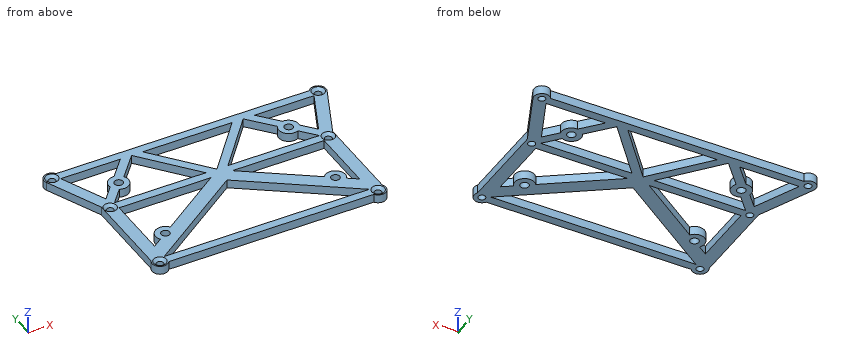
```python
from build123d import *

# Parameters (mm, degrees)
SKETCH1_R           = 1.25
BOSS_EXTRUDE1_DEPTH = 3
CHAMFER1_SIZE       = 1
SKETCH2_R           = 3.5
BOSS_EXTRUDE2_DEPTH = 3
SKETCH2_3_R         = 1.5
CUT_EXTRUDE1_DEPTH  = 3


with BuildPart() as part:
    # Sketch1 → Boss-Extrude1 (new body)
    with BuildSketch(Plane.XY):
        with BuildLine():
            Line((6.173773471, 33.368208058), (-2.509184891, 52.727938114))
            ThreePointArc((-2.509184891, 52.727938114), (-1.316660917, 56.267635348), (2.304886114, 55.353323017))
            Line((2.304886114, 55.353323017), (91.695113886, 55.353323017))
            ThreePointArc((91.695113886, 55.353323017), (95.316660917, 56.267635348), (96.509184891, 52.727938114))
            Line((96.509184891, 52.727938114), (87.826226529, 33.368208058))
            Line((87.826226529, 33.368208058), (87.826226529, 1.466686789))
            ThreePointArc((87.826226529, 1.466686789), (86.983381771, -2.315616229), (83.195113886, -1.5))
            Line((83.195113886, -1.5), (10.804886114, -1.5))
            ThreePointArc((10.804886114, -1.5), (7.016618229, -2.315616229), (6.173773471, 1.466686789))
            Line((6.173773471, 1.466686789), (6.173773471, 33.368208058))
        make_face()
        with Locations((0, 53.853323017)):
            Circle(SKETCH1_R, mode=Mode.SUBTRACT)
        with Locations((8.5, 31.901521269)):
            Circle(SKETCH1_R, mode=Mode.SUBTRACT)
        with Locations((8.5, 0)):
            Circle(SKETCH1_R, mode=Mode.SUBTRACT)
        with Locations(Location((85.5, 0, 0), (0, 0, 180))):
            Circle(SKETCH1_R, mode=Mode.SUBTRACT)
        with Locations(Location((85.5, 31.901521269, 0), (0, 0, 180))):
            Circle(SKETCH1_R, mode=Mode.SUBTRACT)
        with Locations(Location((94, 53.853323017, 0), (0, 0, 180))):
            Circle(SKETCH1_R, mode=Mode.SUBTRACT)
        Polygon((9.452473834, 36.416891788), (2.304886114, 52.353323017), (23.327202938, 52.353323017), align=None, mode=Mode.SUBTRACT)
        Polygon((10.804886114, 33.401521269), (43.095167668, 33.401521269), (27.304886114, 52.353323017), align=None, mode=Mode.SUBTRACT)
        Polygon((10.804886114, 30.401521269), (43.196670996, 30.401521269), (10.804886114, 7.613376738), align=None, mode=Mode.SUBTRACT)
        Polygon((10.804886114, 1.5), (83.195113886, 1.5), (47, 26.963847996), align=None, mode=Mode.SUBTRACT)
        Polygon((83.195113886, 30.401521269), (83.195113886, 7.613376738), (50.803329004, 30.401521269), align=None, mode=Mode.SUBTRACT)
        Polygon((84.547526166, 36.416891788), (91.695113886, 52.353323017), (70.672797062, 52.353323017), align=None, mode=Mode.SUBTRACT)
        Polygon((47, 33.401521269), (31.209718446, 52.353323017), (62.790281554, 52.353323017), align=None, mode=Mode.SUBTRACT)
        Polygon((50.904832332, 33.401521269), (83.195113886, 33.401521269), (66.695113886, 52.353323017), align=None, mode=Mode.SUBTRACT)
    extrude(amount=BOSS_EXTRUDE1_DEPTH)

    # Chamfer1
    chamfer1_edges = [part.edges().sort_by_distance(p)[0] for p in [
        (86.75, 0, 3),
        (86.75, 31.901521269, 3),
        (95.25, 53.853323017, 3),
        (-1.25, 53.853323017, 3),
        (7.25, 31.901521269, 3),
        (7.25, 0, 3),
    ]]
    chamfer(chamfer1_edges, length=CHAMFER1_SIZE)

    # Sketch2 → Boss-Extrude2 (add)
    with BuildSketch(Plane.XY.offset(3)):
        with Locations((17, 41.926661509)):
            Circle(SKETCH2_R)
        with Locations((17, 11.926661509)):
            Circle(SKETCH2_R)
        with Locations((77, 41.926661509)):
            Circle(SKETCH2_R)
        with Locations((77, 11.926661509)):
            Circle(SKETCH2_R)
    extrude(amount=-BOSS_EXTRUDE2_DEPTH)

    # Sketch2<3> → Cut-Extrude1 (cut)
    with BuildSketch(Plane.XY.offset(3)):
        with Locations((17, 11.926661509)):
            Circle(SKETCH2_3_R)
        with Locations((77, 11.926661509)):
            Circle(SKETCH2_3_R)
        with Locations((17, 41.926661509)):
            Circle(SKETCH2_3_R)
        with Locations((77, 41.926661509)):
            Circle(SKETCH2_3_R)
    extrude(amount=-CUT_EXTRUDE1_DEPTH, mode=Mode.SUBTRACT)


solid = part.part
```
Could you check a few things on this model? Use its own coordinates, in mm. Round coordinates to 2 decimals unless told otherwise and drop trailing zeros. Loops run counter-clockwise (first coordinate to the right, second up) from the corner with the lowest first, then second, coordinate; pieces in that order, holes last.
Q1. Please list where these lines run through material, in increasing order: L1, parallel to Y at x = 15, z = 2.8; L2, parallel to X at y = 8.5, z = 1.25; L3, parallel to Y at x = 52.5, z = 1.5.
Q2. I want a section at D-D (x = 29). Write out the boundary of the cut face in (y, z).
Q3. For P1, Ø4, axis at x = 0, y = 53.85, coming from the +Z side; P2, Ø1, axis at y = 36.5, z = 1.5, coming from the +X side; P3, Ø1, axis at x = 47, z = 2.5, coming from the +Y side, each with a flat end and sliding along its axis, tell me the tip position at first contact or that it passes through.
Q4. I want a section at B-B (x = 94). Write out the boundary of the cut face in (y, z).
Q5. I want a section at A-A (y = 0). Write out the boundary of the cut face in (x, z), and give its area (4 significant figures).
Q6. I want a section at C-C (x = 39.5). Write out the boundary of the cut face in (y, z), and give its area (3 significant figures).
Answer below:
1. L1: y = -1.5 to 1.5, 4.45 to 14.8, 30.4 to 33.4, 38.22 to 44.8, 52.35 to 55.35
1. L2: x = 6.17 to 10.8, 12.07 to 20.75, 73.25 to 81.93, 83.2 to 87.83
1. L3: y = -1.5 to 1.5, 23.09 to 29.21, 30.4 to 33.4, 35.32 to 40, 52.35 to 55.35
2. outline: (-1.5, 0) - (1.5, 0) - (1.5, 3) - (-1.5, 3) - close; (14.3, 0) - (20.41, 0) - (20.41, 3) - (14.3, 3) - close; (30.4, 0) - (33.4, 0) - (33.4, 3) - (30.4, 3) - close; (50.32, 0) - (55.35, 0) - (55.35, 3) - (50.32, 3) - close
3. P1: stops at z = 2.75
3. P2: stops at x = 89.46
3. P3: stops at y = 55.35
4. outline: (47.13, 0) - (52.6, 0) - (52.6, 2) - (51.6, 3) - (47.13, 3) - close; (55.1, 0) - (56.6, 0) - (56.6, 3) - (56.1, 3) - (55.1, 2) - close
5. outline: (5.75, 0) - (7.25, 0) - (7.25, 2) - (6.25, 3) - (5.75, 3) - close; (9.75, 0) - (84.25, 0) - (84.25, 2) - (83.25, 3) - (10.75, 3) - (9.75, 2) - close; (86.75, 0) - (88.25, 0) - (88.25, 3) - (87.75, 3) - (86.75, 2) - close
5. area: 230.5 mm2
6. outline: (-1.5, 0) - (1.5, 0) - (1.5, 3) - (-1.5, 3) - close; (21.69, 0) - (27.8, 0) - (27.8, 3) - (21.69, 3) - close; (30.4, 0) - (33.4, 0) - (33.4, 3) - (30.4, 3) - close; (37.72, 0) - (42.4, 0) - (42.4, 3) - (37.72, 3) - close; (52.35, 0) - (55.35, 0) - (55.35, 3) - (52.35, 3) - close
6. area: 59.4 mm2
